Here's how the part is built. I have some questions about the finished solid (model axes, mm). Face numbers are marked on the shaded views. Coordinates: 2 decimals unless noted, no trailing zeros. Write each loop counter-clockwise with the first axis right and the second up, starting at its lowest first coordinate (ties: lowest second). Pieces come first, ordered by that corner, then holes.
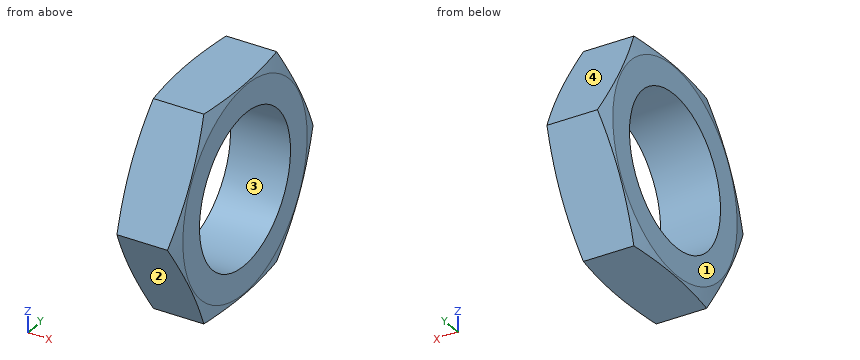
Autodesk Inventor part; units mm, degrees
ref_plane "IP_Holder_XY" through (0, 0, 0) normal (-1, 0, 0) x (0, 0, -1)
ref_plane "IP_Holder_YZ" through (0, 0, 0) normal (0, 0, -1) x (0, -1, 0)
ref_plane "IP_Holder_ZX" through (0, 0, 0) normal (0, -1, 0) x (-1, 0, 0)
sketch "Sketch_1" plane through (0, 0, 0) normal (0, 0, 1) x (1, 0, 0)
  line L0 (4, 0) -> (0, 0)
  line L1 (0, 0) -> (0, 6.9)
  line L2 (0, 6.9) -> (0.3698, 8.28)
  line L3 (0.3698, 8.28) -> (3.6302, 8.28)
  line L4 (3.6302, 8.28) -> (4, 6.9)
  line L5 (4, 6.9) -> (4, 0)
  line L6 (4, 0) -> (0, 0)
revolve "Revolution1" add sketch "Sketch_1" angle 360 about axis through (4, 0, 0) along (1, 0, 0)
sketch "Sketch2" plane through (0, 0, 0) normal (-1, 0, 0) x (0, 0, 1)
  point P0 (0, 0)
hole "Hole1" at (0, 0, 0) direction (1, 0, 0) diameter 10.106 depth 4
sketch "Sketch_3" plane through (0, 0, 0) normal (1, 0, 0) x (0, 1, 0)
  line L0 (14, 14) -> (-14, 14)
  line L1 (-14, 14) -> (-14, -14)
  line L2 (-14, -14) -> (14, -14)
  line L3 (14, -14) -> (14, 14)
  line L4 (-4.0415, 7) -> (-8.0829, 0)
  line L5 (-8.0829, 0) -> (-4.0415, -7)
  line L6 (-4.0415, -7) -> (4.0415, -7)
  line L7 (4.0415, -7) -> (8.0829, 0)
  line L8 (8.0829, 0) -> (4.0415, 7)
  line L9 (4.0415, 7) -> (-4.0415, 7)
extrude "Extrusion1" cut sketch "Sketch_3" along normal blind 4
ref_plane "IP_Holder_XY" through (0, 0, 0) normal (-1, 0, 0) x (0, 0, -1)
ref_plane "IP_Holder_YZ" through (0, 0, 0) normal (0, 0, -1) x (0, -1, 0)
ref_plane "IP_Holder_ZX" through (0, 0, 0) normal (0, -1, 0) x (-1, 0, 0)
properties part number "MN12P1(MNF12P1)"
1) Imagine slicing it at A-A on y = 0. Please give me the cut outline in (x, z), then the cut area to 3 significant figures.
Values follow:
outline: (0, -6.9) - (0.03, -7) - (3.97, -7) - (4, -6.9) - (4, -5.05) - (0, -5.05) - close; (0, 5.05) - (4, 5.05) - (4, 6.9) - (3.97, 7) - (0.03, 7) - (0, 6.9) - close
area: 15.6 mm2
2) Will these pins go through, and if not, where does the flat tip stop? pin 1 (2 mm diameter, centred on y = -5.5, z = 1.5, fed in from -X); pin 2 (1.5 mm diameter, centred on x = 2, z = -2.5, fed in from +Y); pin 3 (1.5 mm diameter, centred on x = 2.5, z = 3.5, fed in from +Y).
Values follow:
pin 1: stops at x = 0
pin 2: stops at y = 7.07
pin 3: stops at y = 6.5
3) I need wall thicknesses on probe 1 along Z at (x, y) = (3, 0); probe 2 along Z at (x, y) = (2.8, -1); probe 3 along Y at (x, z) = (1, -2.5). Which ranges of each line are inside material? Lowest first, please.
Values follow:
probe 1: z = -7 to -5.05, 5.05 to 7
probe 2: z = -7 to -4.95, 4.95 to 7
probe 3: y = -6.64 to -4.39, 4.39 to 6.64
4) We'd pull the mould along Y, two halves only. Please class the marked faces 1, 2, 3 and 4: pulls with the +Y half, pulls with the -Y half, needs draft (parallel to the pull), parting line crosses it, or undercut.
Values follow:
face 1: needs draft
face 2: pulls with the -Y half
face 3: undercut
face 4: pulls with the +Y half
